```python
from build123d import *

# Parameters (mm, degrees)
F0_W     = 139.7
F0_H     = 51.308
F1_DEPTH = 6.35
F2_R     = 1.27
F3_DEPTH = 10.414
F2_R_2   = 3.175
F4_DEPTH = 2.54
F5_DEPTH = 7.112


with BuildPart() as f1:
    # F0 (on Top) → F1 (new body)
    with BuildSketch(Plane.XY):
        with Locations((18.3706976533, 5.599814237)):
            Rectangle(F0_W, F0_H)
    extrude(amount=F1_DEPTH)

    # F2 (on face) → F3 (cut)
    with BuildSketch(Plane.XY.offset(6.35)):
        with BuildLine():
            ThreePointArc((-43.8593023467, 5.599814237), (-45.1293023467, 6.869814237), (-46.3993023467, 5.599814237))
            ThreePointArc((-46.3993023467, 5.599814237), (-45.1293023467, 4.329814237), (-43.8593023467, 5.599814237))
        make_face()
        with Locations((81.8706976533, 5.599814237)):
            Circle(F2_R)
    extrude(amount=-F3_DEPTH, mode=Mode.SUBTRACT)

    # F2 (on face) → F4 (cut)
    with BuildSketch(Plane.XY.offset(6.35)):
        with BuildLine():
            ThreePointArc((-41.9543023467, 5.599814237), (-45.1293023467, 8.774814237), (-48.3043023467, 5.599814237))
            ThreePointArc((-48.3043023467, 5.599814237), (-45.1293023467, 2.424814237), (-41.9543023467, 5.599814237))
        make_face()
        with BuildLine():
            ThreePointArc((-43.8593023467, 5.599814237), (-45.1293023467, 4.329814237), (-46.3993023467, 5.599814237))
            ThreePointArc((-46.3993023467, 5.599814237), (-45.1293023467, 6.869814237), (-43.8593023467, 5.599814237))
        make_face(mode=Mode.SUBTRACT)
        with Locations((81.8706976533, 5.599814237)):
            Circle(F2_R_2)
        with Locations((81.8706976533, 5.599814237)):
            Circle(F2_R, mode=Mode.SUBTRACT)
    extrude(amount=-F4_DEPTH, mode=Mode.SUBTRACT)

    # F5 (add): faces of the model
    f5_faces = [f1.faces().sort_by_distance(p)[0] for p in [
        (-42.0441049079, 5.599814237, 3.81),
        (78.7855002145, 5.599814237, 3.81),
    ]]
    extrude(f5_faces, amount=-F5_DEPTH)


solid = f1.part
```
For this review, take the finished solid that the model builds, in its own axes (mm). A direction names the side the tool comes from. Round coordinates to 2 decimals unless told otherwise and drop trailing zeros. Write each loop counter-clockwise with the first axis right and the second up, starting at its lowest first coordinate (ties: lowest second). Pieces come first, ordered by that corner, then holes. Notation, with made-up numbers: (81, -1.5) - (118, -1.5) arc R29 cw to (118, 20.5) - close; hole circle Ø3 at (-32.75, -20). An arc over 180 degrees is marked (long way). Write each question's results on one line, items separated by ' | '.
Item 1: For faces 1 (the face through (-45, 4, 3.81)), 2 (the face through (-45, 4, -3.302)), 3 (the face through (-44.72, 2.45, -1.63)), list the 3-axis set-ups (+Z, -Z, +X, -X, +Y, -Y) from which the entire face can be reached by the end or side of a thin tool; tool diameter is ignored.
Calculated:
face 1: +Z | face 2: -Z, +X, -X, +Y, -Y | face 3: -Z
Item 2: Take a section at A-A on z = -1.25. State the section outline as (x, y) points (3 decimals), then the cut area to 3 significant figures.
Calculated:
outline: circle Ø6.35 at (-45.129, 5.6); circle Ø6.35 at (81.871, 5.6); hole circle Ø2.54 at (-45.129, 5.6); hole circle Ø2.54 at (81.871, 5.6) | area: 53.2 mm^2
Item 3: Draft analysis for pull direction X (two halves, no side actions). For faces 4 (the face through (78.7, 5.74, 5.1)), 5 (the face through (-44.72, 2.45, 5.1)), 6 (the face through (82, 4, -3.302)), 7 (the face through (88.221, 5, 3)), state which applies: pulls with the +X half, pulls with the -X half, needs draft (parallel to the pull), parting line crosses it, or undercut.
Calculated:
face 4: undercut | face 5: undercut | face 6: needs draft | face 7: pulls with the +X half
Item 4: To check wall thickness, follow line 1 along Z through (x, y) = (25, -12.5). State the ranges of the line that lie inside material, in increasing order. Write a range as from..to.
Calculated:
line 1: z = 0..6.35
Item 5: Take a section at C-C on y = 11.5. State the section outline as (x, z) points, then the cut area to 3 significant figures.
Calculated:
outline: (-51.48, 0) - (88.22, 0) - (88.22, 6.35) - (-51.48, 6.35) - close | area: 887 mm^2
Item 6: For pin 1 (3 mm diameter, centred on x = 82, y = 5.5, fed in from +Z); pin 2 (12 mm diameter, centred on x = 7.5, y = 4.5, fed in from -Z), all flat-tipped, find the tip position at first contact; note any pin that passes through.
Calculated:
pin 1: stops at z = 3.81 | pin 2: stops at z = 0
Item 7: Take a section at B-B on x = 11.5. State the section outline as (y, z) points.
Calculated:
outline: (-20.05, 0) - (31.25, 0) - (31.25, 6.35) - (-20.05, 6.35) - close
